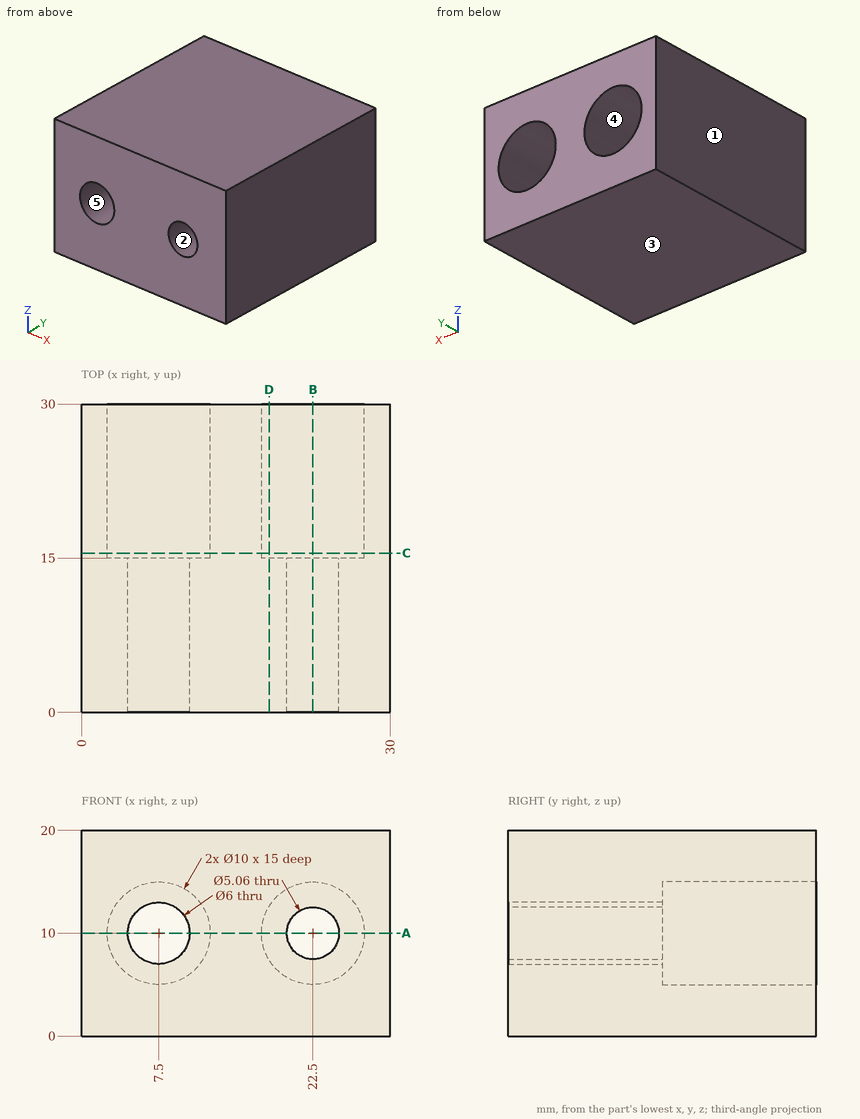
Could you check a few things on this drawing? It's one solid part, dimensions in mm from its lowest x, y, z. A direction names the side the tool comes from. Round coordinates to 2 decimals unless told otherwise and drop trailing zeros. Order: outer loops, then holes, each group sorted by start corner. A loop starts at its lowest first (then second) coordinate and runs counter-clockwise, first axis right, second up. Notation, with made-up numbers: M 34.25,54 L 49.25,54 A14 cw 49.25,76 Z; hole C 76.5,11.5 d11. An arc over 180 degrees is marked long. Return JSON: item names as keys, results as strings. Group by question number.
1. Please list where these lines run through material, in increasing order: probe 1 along X at (y, z) = (5, 10); probe 2 along X at (y, z) = (23.25, 10); probe 3 along Y at (x, z) = (23.25, 6.5).
2. If we section it at D-D on x = 18.25: List the corners of the cut face in (y, z) for me.
3. I'm going to push a flat-ended pin straight in: pin 1 Ø9 at (x, z) = (22.5, 10) entering from +Y. Where does the tip first touch, or does it pass through?
4. If we section it at A-A on z = 10: List the corners of the cut face in (x, y) for me.
5. If we section it at B-B on x = 22.5: List the corners of the cut face in (y, z) for me.
6. If we mould it in two halves opening along Z, with no side actions, what happens to the marked faces 1, 2 and 3? For each: pulls with the +Z half, pulls with the -Z half, needs draft (parallel to the pull), parting line crosses it, or undercut.
7. If we section it at C-C on y = 15.5: List the corners of the cut face in (x, z) for me.
8. On a 3-axis mill with a long thin cutter (end or side, diameter ignored), from which of +Z, -Z, +X, -X, +Y, -Y can I reach the whole of each face in a straight line? I mean the marked faces 4 and 5. Say none if no direction works.
Reply:
{
 "1": {"probe 1": "0 to 4.5, 10.5 to 19.97, 25.03 to 30", "probe 2": "0 to 2.5, 12.5 to 17.5, 27.5 to 30", "probe 3": "0 to 15"},
 "2": {"outline": "M 0,0 L 30,0 L 30,7.37 L 15,7.37 L 15,12.63 L 30,12.63 L 30,20 L 0,20 Z"},
 "3": {"pin 1": "y = 15"},
 "4": {"outline": "M 0,0 L 4.5,0 L 4.5,15 L 2.5,15 L 2.5,30 L 0,30 Z; M 10.5,0 L 19.97,0 L 19.97,15 L 17.5,15 L 17.5,30 L 12.5,30 L 12.5,15 L 10.5,15 Z; M 25.03,0 L 30,0 L 30,30 L 27.5,30 L 27.5,15 L 25.03,15 Z"},
 "5": {"outline": "M 0,0 L 30,0 L 30,5 L 15,5 L 15,7.47 L 0,7.47 Z; M 0,12.53 L 15,12.53 L 15,15 L 30,15 L 30,20 L 0,20 Z"},
 "6": {"face 1": "needs draft", "face 2": "undercut", "face 3": "pulls with the -Z half"},
 "7": {"outline": "M 0,0 L 30,0 L 30,20 L 0,20 Z; hole C 7.5,10 d10; hole C 22.5,10 d10"},
 "8": {"face 4": "+Y", "face 5": "+Y, -Y"}
}
